from build123d import *

# Parameters (mm, degrees)
SKETCH1_R   = 6.35
SKETCH1_R_2 = 3.175
BORE_DEPTH  = 4.7625
FILLET_2_R  = 0.47625


with BuildPart() as part:
    # Sketch1 → Bore (new body)
    with BuildSketch(Plane(origin=(0, 0, 0), x_dir=(1, 0, 0), z_dir=(0, 1, 0))):
        Circle(SKETCH1_R)
        Circle(SKETCH1_R_2, mode=Mode.SUBTRACT)
    extrude(amount=BORE_DEPTH)

    # Fillet 2
    fillet_2_edges = [part.edges().sort_by_distance(p)[0] for p in [
        (-6.35, 0, 0),
        (-6.35, 4.7625, 0),
        (-3.175, 0, 0),
        (-3.175, 4.7625, 0),
    ]]
    fillet(fillet_2_edges, radius=FILLET_2_R)


solid = part.part
The model under review builds one solid part; all positions refer to its coordinate system, in mm. Round coordinates to 2 decimals unless told otherwise and drop trailing zeros. Write each loop counter-clockwise with the first axis right and the second up, starting at its lowest first coordinate (ties: lowest second). Pieces come first, ordered by that corner, then holes. Notation, with made-up numbers: M 61,-28 L 83,-28 A33 cw 83,8 Z; hole C 88.5,50 d5. An arc over 180 degrees is marked long. Use a Markdown table: item, result. Add a question column.
Q1. To check wall thickness, follow line 1 (Z direction, x = 0, y = 2.7) (3 decimals); line 2 (X direction, y = 1.6, z = 0.5). State the ranges of each line that lie inside material, in increasing order.
Q2. The part is to be moulded in two halves that separate along X. For faces 1 (the face through (3, 0, -3)), 2 (the face through (-1.38, 2.35, 6.2)), 3 (the face through (-0.69, 2.35, 3.1)), say which applies: pulls with the +X half, pulls with the -X half, needs draft (parallel to the pull), parting line crosses it, or undercut.
Q3. Insertion check: pin 1 (1 mm diameter, centred on y = 0.5, z = -3.5, fed in from +X). The pin has a flat end and moves straight along its axis. Give the tip position at first contact, or say it passes through.
Q4. We need section C-C, the plane y = 4. State the section outline as (x, z) points (3 decimals).
Findings below:
| question | item | result |
|---|---|---|
| 1 | line 1 | z = -6.35 to -3.175, 3.175 to 6.35 |
| 1 | line 2 | x = -6.33 to -3.14, 3.14 to 6.33 |
| 2 | face 1 | needs draft |
| 2 | face 2 | parting line crosses it |
| 2 | face 3 | undercut |
| 3 | pin 1 | stops at x = 5.6 |
| 4 | outline | C 0,0 d12.7; hole C 0,0 d6.35 |
